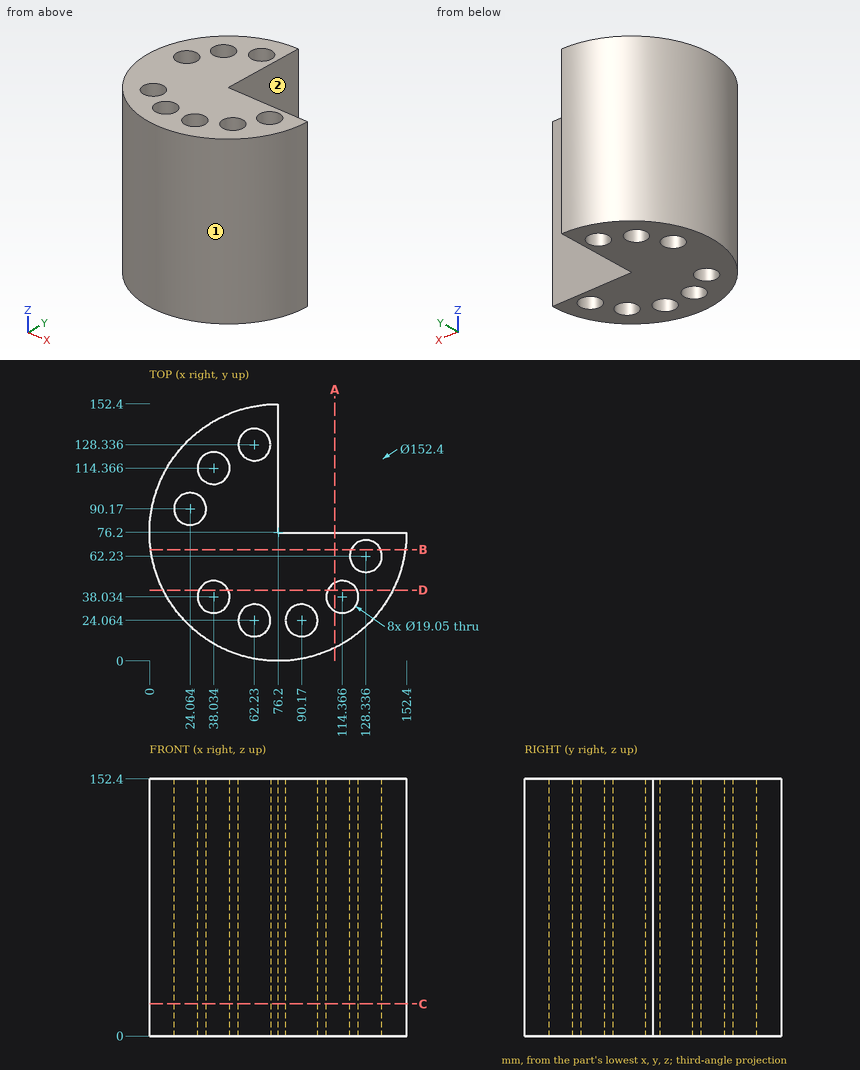
The drawing under review shows one solid part. Ordinate dimensions are in mm from its lowest x, y, z. A direction names the side the tool comes from. Give positions to 0.01 mm unless a question says otherwise; leave off trailing zeros. Order: outer loops, then holes, each group sorted by start corner. A loop starts at its lowest first (then second) coordinate and runs counter-clockwise, first axis right, second up. Notation, with made-up numbers: (-12.75, -27.75) - (17.25, -27.75) arc R31 ccw to (17.25, -3.75) - close; hole circle Ø3 at (55, -29.5). An arc over 180 degrees is marked (long way). Answer as a JSON object with one key per item and string values. Group by question number.
Item 1: Clearance check with flat-ended pins moving along their axes: pin 1 Ø17 at (x, y) = (90.17, 24.06) entering from -Z; pin 2 Ø6 at (x, z) = (87, 93) entering from -Y; pin 3 Ø4 at (y, z) = (88, 111.5) entering from -X; pin 4 Ø23 at (y, z) = (123, 105) entering from +X. State where each tip first meets the part, or that it passes through.
Item 2: Take a section at B-B on y = 66. Give the boundary of the cut face in (x, z).
Item 3: Take a section at C-C on z = 19. Give the number of separate pieces and of enclosed holes in the cut face, and give its area (3 significant figures).
Item 4: Wall thickness on line 1 along Y through (x, z) = (55.5, 82) (1 decimal); line 2 along X through (y, z) = (98, 138.5) (1 decimal); line 3 along Y through (x, z) = (67, 36.5): over which ranges is each line inside the solid? List them lowest first.
Item 5: Take a section at D-D on y = 42. Give the boundary of the cut face in (x, z), and give its area (3 significant figures).
Item 6: Take a section at A-A on x = 110. Give the boundary of the cut face in (y, z).
Item 7: Machinability: for the marked faces 1 and 2, which of the approach directions +Z, -Z, +X, -X, +Y, -Y give a long, thin tool a straight path to every point of the face, cutting with its end or side? Answer none if there is none.
Reported:
{
 "1": {"pin 1": "through", "pin 2": "y = 0.4", "pin 3": "x = 0.63", "pin 4": "x = 76.2"},
 "2": {"outline": "(0.69, 0) - (119.59, 0) - (119.59, 152.4) - (0.69, 152.4) - close; (137.08, 0) - (151.71, 0) - (151.71, 152.4) - (137.08, 152.4) - close"},
 "3": {"separate pieces": "1", "enclosed holes": "8", "area": "11,400 mm^2"},
 "4": {"line 1": "2.9 to 17.3, 30.8 to 121.6, 135.1 to 149.5", "line 2": "3.2 to 18.6, 29.5 to 76.2", "line 3": "0.56 to 15.82, 32.31 to 120.09, 136.58 to 151.84"},
 "5": {"outline": "(8.11, 0) - (29.37, 0) - (29.37, 152.4) - (8.11, 152.4) - close; (46.69, 0) - (105.71, 0) - (105.71, 152.4) - (46.69, 152.4) - close; (123.03, 0) - (144.29, 0) - (144.29, 152.4) - (123.03, 152.4) - close", "area": "15,500 mm^2"},
 "6": {"outline": "(7.91, 0) - (29.57, 0) - (29.57, 152.4) - (7.91, 152.4) - close; (46.5, 0) - (76.2, 0) - (76.2, 152.4) - (46.5, 152.4) - close"},
 "7": {"face 1": "+Z, -Z", "face 2": "+Z, -Z, +X, +Y"}
}
